Read the model definition and answer for the solid it produces. Units are mm, in the model's axes. A direction names the side the tool comes from. Coordinates: 2 decimals unless noted, no trailing zeros. Order: outer loops, then holes, each group sorted by start corner. A loop starts at its lowest first (then second) coordinate and runs counter-clockwise, first axis right, second up. Notation, with made-up numbers: (-23, -13) - (-8, -13) arc R14 cw to (-8, -9) - close; hole circle Ø7 at (22.5, -8). An arc over 180 degrees is marked (long way). Write item = value, one per line.
from build123d import *

# Parameters (mm, degrees)
ESBO_O2_W                = 85
ESBO_O2_H                = 35
RESSALTO_EXTRUS_O2_DEPTH = 3
FURO_COM_FOLGA_DE_M41_D  = 4.8
ESBO_O10_W               = 3.01
ESBO_O10_H               = 8.01
CORTE_EXTRUS_O2_DEPTH    = 10
ESBO_O11_W               = 3
ESBO_O11_H               = 0.25
ESBO_O11_W_2             = 0.25
ESBO_O11_H_2             = 3.603257419
CORTE_EXTRUS_O3_DEPTH    = 47.059743812


with BuildPart() as part:
    # Esboço2 → Ressalto-extrusão2 (new body)
    with BuildSketch(Plane(origin=(0, 0, 0), x_dir=(1, 0, 0), z_dir=(0, 1, 0))):
        Rectangle(ESBO_O2_W, ESBO_O2_H)
    extrude(amount=RESSALTO_EXTRUS_O2_DEPTH)

    # Furo com folga de M41 (through all)
    with Locations(Plane(origin=(0, 0, 0), x_dir=(-1, 0, 0), z_dir=(0, -1, 0))):
        with Locations((30, -11.5), (30, 11.5), (-30, 11.5), (-30, -11.5)):
            Hole(FURO_COM_FOLGA_DE_M41_D / 2)

    # Esboço10 → Corte-extrusão2 (cut)
    with BuildSketch(Plane(origin=(0, 3, 0), x_dir=(1, 0, 0), z_dir=(0, 1, 0))):
        with Locations((-37.995, 10.005)):
            Rectangle(ESBO_O10_W, ESBO_O10_H)
        with Locations((-37.995, -10.005)):
            Rectangle(ESBO_O10_W, ESBO_O10_H)
        with Locations((37.995, -10.005)):
            Rectangle(ESBO_O10_W, ESBO_O10_H)
        with Locations((37.995, 10.005)):
            Rectangle(ESBO_O10_W, ESBO_O10_H)
    extrude(amount=-CORTE_EXTRUS_O2_DEPTH, mode=Mode.SUBTRACT)

    # Esboço11 → Corte-extrusão3 (cut, through all)
    with BuildSketch(Plane(origin=(0, 3, 0), x_dir=(1, 0, 0), z_dir=(0, 1, 0))):
        with Locations((-41, 10.005)):
            Rectangle(ESBO_O11_W, ESBO_O11_H)
        with Locations((-30, 15.698371291)):
            Rectangle(ESBO_O11_W_2, ESBO_O11_H_2)
        with Locations((-30, -15.698371291)):
            Rectangle(ESBO_O11_W_2, ESBO_O11_H_2)
        with Locations((-41, -10.005)):
            Rectangle(ESBO_O11_W, ESBO_O11_H)
        with Locations((41, -10.005)):
            Rectangle(ESBO_O11_W, ESBO_O11_H)
        with Locations((30, -15.698371291)):
            Rectangle(ESBO_O11_W_2, ESBO_O11_H_2)
        with Locations((30, 15.698371291)):
            Rectangle(ESBO_O11_W_2, ESBO_O11_H_2)
        with Locations((41, 10.005)):
            Rectangle(ESBO_O11_W, ESBO_O11_H)
    extrude(amount=-CORTE_EXTRUS_O3_DEPTH, mode=Mode.SUBTRACT)


solid = part.part
1) For faces 1 (the face through (41, 2, -10.13)), 2 (the face through (42.5, 1, 0)), 3 (the face through (-41, 2, -9.88)), 4 (the face through (-38, 2, -6)), 5 (the face through (-29.875, 2, -16)), determine the directions among +Z, -Z, +X, -X, +Y, -Y from which every point of the face is accessible in a straight line to the end or side of a thin tool.
Returned:
face_1 = +X, +Y, -Y
face_2 = +Z, -Z, +X, +Y, -Y
face_3 = -X, +Y, -Y
face_4 = +Y, -Y
face_5 = -Z, +Y, -Y
2) The part is cut by section A-A (z = 7). Determine the outline of the cut face in (x, y), and give its area (3 significant figures).
Returned:
outline = (-42.5, 0) - (-39.5, 0) - (-39.5, 3) - (-42.5, 3) - close; (-36.49, 0) - (36.49, 0) - (36.49, 3) - (-36.49, 3) - close; (39.5, 0) - (42.5, 0) - (42.5, 3) - (39.5, 3) - close
area = 237 mm^2
3) Determine the mould class of faces 6 (the face through (38, 2, 14.01)), 7 (the face through (-36, 1, 17.5)), 8 (the face through (29.875, 2, -16)) for opening direction Z: pulls with the +Z half, pulls with the -Z half, needs draft (parallel to the pull), parting line crosses it, or undercut.
Returned:
face_6 = undercut
face_7 = pulls with the +Z half
face_8 = needs draft
4) Flat-ended cylindrical pins translate along their axes: pin 1 Ø1.5 at (y, z) = (1, 10) entering from +X; pin 2 Ø4.5 at (x, z) = (-30, 11.5) entering from -Y. Find the tip coordinate at first contact, or state that the pin passes through.
Returned:
pin_1 = 42.5
pin_2 = through
5) Straight lines are drawn through the part: line 1 along X through (y, z) = (1.1, 11.5); line 2 along Z through (x, y) = (-38, 2.6); line 3 along Z through (x, y) = (31, 2.25). For each, find the intervals that lie inside material, in ascending order. Write a range as from..to.
Returned:
line_1 = -42.5..-39.5, -36.49..-32.4, -27.6..27.6, 32.4..36.49, 39.5..42.5
line_2 = -17.5..-14.01, -6..6, 14.01..17.5
line_3 = -17.5..-13.68, -9.32..9.32, 13.68..17.5
6) The part is cut by section B-B (x = 29). Determine the outline of the cut face in (y, z), and give its area (3 significant figures).
Returned:
outline = (0, -17.5) - (3, -17.5) - (3, -13.68) - (0, -13.68) - close; (0, -9.32) - (3, -9.32) - (3, 9.32) - (0, 9.32) - close; (0, 13.68) - (3, 13.68) - (3, 17.5) - (0, 17.5) - close
area = 78.8 mm^2
